Model file for the job. Use its own axes, mm. Round coordinates to 2 decimals unless told otherwise and drop trailing zeros. Use a Markdown table: item, result. Add a question column.
Q1. Cut at A-A (x = -32). State how many separate pieces and enclosed holes the cut face has, plus the area to 3 significant figures.
Q2. Pin check, flat tips, straight feed: pin 1 (0.6 mm diameter, centred on x = -60.5, y = 0.5, fed in from -Z) (3 decimals); pin 2 (0.5 mm diameter, centred on x = -20.5, y = -0.5, fed in from -Z); pin 3 (1 mm diameter, centred on y = -0.5, z = 17.5, fed in from -X). Stop position of each tip, or through.
Q3. Probe line 1 (X direction, y = 0.2, z = 0); line 2 (Z direction, x = -20.5, y = -1.8); line 3 (X direction, y = -1.55, z = 3.5). List the from-to ranges inside material, lowest first. Write a range as from..to.
from build123d import *

# Parameters (mm, degrees)
SKETCH1_R           = 12.7
BOSS_EXTRUDE1_DEPTH = 2.38125
CUT_EXTRUDE1_DEPTH  = 83.900304501
FILLET1_R           = 3.175
SKETCH3_RX          = 21.59
SKETCH3_RY          = 20.32
CUT_EXTRUDE2_DEPTH  = 83.900304501
CIRPATTERN1_COUNT   = 6
SKETCH4_R           = 1.27
CUT_EXTRUDE3_DEPTH  = 83.900304648
CIRPATTERN2_COUNT   = 6
BOSS_EXTRUDE2_DEPTH = 4.7625


with BuildPart() as part:
    # Sketch1 → Boss-Extrude1 (new, symmetric)
    with BuildSketch(Plane(origin=(0, 0, 0), x_dir=(1, 0, 0), z_dir=(0, 1, 0))):
        with BuildLine():
            Line((-60.1472, 5.553404471), (-60.1472, 9.525))
            Line((-60.1472, 9.525), (-38.322491971, 47.326503167))
            Line((-38.322491971, 47.326503167), (-34.88298935, 49.312300931))
            ThreePointArc((-34.88298935, 49.312300931), (-27.384375, 47.431128834), (-25.26421065, 54.865705402))
            Line((-25.26421065, 54.865705402), (-21.824708029, 56.851503167))
            Line((-21.824708029, 56.851503167), (21.824708029, 56.851503167))
            Line((21.824708029, 56.851503167), (25.26421065, 54.865705402))
            ThreePointArc((25.26421065, 54.865705402), (27.384375, 47.431128834), (34.88298935, 49.312300931))
            Line((34.88298935, 49.312300931), (38.322491971, 47.326503167))
            Line((38.322491971, 47.326503167), (60.1472, 9.525))
            Line((60.1472, 9.525), (60.1472, 5.553404471))
            ThreePointArc((60.1472, 5.553404471), (54.76875, 0), (60.1472, -5.553404471))
            Line((60.1472, -5.553404471), (60.1472, -9.525))
            Line((60.1472, -9.525), (38.322491971, -47.326503167))
            Line((38.322491971, -47.326503167), (34.88298935, -49.312300931))
            ThreePointArc((34.88298935, -49.312300931), (27.384375, -47.431128834), (25.26421065, -54.865705402))
            Line((25.26421065, -54.865705402), (21.824708029, -56.851503167))
            Line((21.824708029, -56.851503167), (-21.824708029, -56.851503167))
            Line((-21.824708029, -56.851503167), (-25.26421065, -54.865705402))
            ThreePointArc((-25.26421065, -54.865705402), (-27.384375, -47.431128834), (-34.88298935, -49.312300931))
            Line((-34.88298935, -49.312300931), (-38.322491971, -47.326503167))
            Line((-38.322491971, -47.326503167), (-60.1472, -9.525))
            Line((-60.1472, -9.525), (-60.1472, -5.553404471))
            ThreePointArc((-60.1472, -5.553404471), (-54.76875, 0), (-60.1472, 5.553404471))
        make_face()
        with Locations(Location((0, 0, 0), (0, 0, 90))):
            Circle(SKETCH1_R, mode=Mode.SUBTRACT)
    extrude(amount=BOSS_EXTRUDE1_DEPTH, both=True)

    # Sketch2 → Cut-Extrude1 (cut, through all)
    with BuildSketch(Plane(origin=(0, 2.38125, 0), x_dir=(1, 0, 0), z_dir=(0, 1, 0))):
        Polygon((10.61724051, -18.3896), (21.234481021, 0), (10.61724051, 18.3896), (-10.61724051, 18.3896), (-21.234481021, 0), (-10.61724051, -18.3896), align=None)
    extrude(amount=-CUT_EXTRUDE1_DEPTH, mode=Mode.SUBTRACT)

    # Fillet1
    fillet1_edges = [part.edges().sort_by_distance(p)[0] for p in [
        (10.61724051, 0, 18.3896),
        (-10.61724051, 0, 18.3896),
        (-21.234481021, 0, 0),
        (-10.61724051, 0, -18.3896),
        (10.61724051, 0, -18.3896),
        (21.234481021, 0, 0),
    ]]
    fillet(fillet1_edges, radius=FILLET1_R)

    # Sketch3 → Cut-Extrude2 (cut, through all)
    with BuildSketch(Plane(origin=(0, 2.38125, 0), x_dir=(1, 0, 0), z_dir=(0, 1, 0))):
        with Locations(Location((0, -56.851503167), (0, 0, -90))):
            Ellipse(SKETCH3_RX, SKETCH3_RY)
    cut_extrude2 = extrude(amount=-CUT_EXTRUDE2_DEPTH, mode=Mode.SUBTRACT)

    # CirPattern1: Cut-Extrude2 ×6 about axis
    cirpattern1_axis = Axis((0, -55, 0), (0, 1, 0))
    for i in range(1, CIRPATTERN1_COUNT):
        add(cut_extrude2.rotate(cirpattern1_axis, i * 360 / CIRPATTERN1_COUNT), mode=Mode.SUBTRACT)

    # Sketch4 → Cut-Extrude3 (cut, through all)
    with BuildSketch(Plane(origin=(0, 2.38125, 0), x_dir=(1, 0, 0), z_dir=(0, 1, 0))):
        with Locations(Location((45.212, 0, 0), (0, 0, 270))):
            Circle(SKETCH4_R)
    cut_extrude3 = extrude(amount=-CUT_EXTRUDE3_DEPTH, mode=Mode.SUBTRACT)

    # CirPattern2: Cut-Extrude3 ×6 about axis
    cirpattern2_axis = Axis((0, 0, 0), (0, 1, 0))
    for i in range(1, CIRPATTERN2_COUNT):
        add(cut_extrude3.rotate(cirpattern2_axis, i * 360 / CIRPATTERN2_COUNT), mode=Mode.SUBTRACT)

    # Sketch6 → Boss-Extrude2 (add)
    # profile 1 of 7: a face of its own
    with BuildSketch(Plane(origin=(0, 2.38125, 0), x_dir=(1, 0, 0), z_dir=(0, 1, 0))):
        with BuildLine():
            Line((11.533784063, -16.8021), (20.317937468, -1.5875))
            ThreePointArc((20.317937468, -1.5875), (20.743306811, 0), (20.317937468, 1.5875))
            Line((20.317937468, 1.5875), (11.533784063, 16.8021))
            ThreePointArc((11.533784063, 16.8021), (10.371653406, 17.964230657), (8.784153406, 18.3896))
            Line((8.784153406, 18.3896), (-8.784153406, 18.3896))
            ThreePointArc((-8.784153406, 18.3896), (-10.371653406, 17.964230657), (-11.533784063, 16.8021))
            Line((-11.533784063, 16.8021), (-20.317937468, 1.5875))
            ThreePointArc((-20.317937468, 1.5875), (-20.743306811, 0), (-20.317937468, -1.5875))
            Line((-20.317937468, -1.5875), (-11.533784063, -16.8021))
            ThreePointArc((-11.533784063, -16.8021), (-10.371653406, -17.964230657), (-8.784153406, -18.3896))
            Line((-8.784153406, -18.3896), (8.784153406, -18.3896))
            ThreePointArc((8.784153406, -18.3896), (10.371653406, -17.964230657), (11.533784063, -16.8021))
        make_face()
        with BuildLine():
            Line((19.658026111, 1.2065), (10.873872705, 16.4211))
            ThreePointArc((10.873872705, 16.4211), (9.990653406, 17.304319299), (8.784153406, 17.6276))
            Line((8.784153406, 17.6276), (-8.784153406, 17.6276))
            ThreePointArc((-8.784153406, 17.6276), (-9.990653406, 17.304319299), (-10.873872705, 16.4211))
            Line((-10.873872705, 16.4211), (-19.658026111, 1.2065))
            ThreePointArc((-19.658026111, 1.2065), (-19.981306811, 0), (-19.658026111, -1.2065))
            Line((-19.658026111, -1.2065), (-10.873872705, -16.4211))
            ThreePointArc((-10.873872705, -16.4211), (-9.990653406, -17.304319299), (-8.784153406, -17.6276))
            Line((-8.784153406, -17.6276), (8.784153406, -17.6276))
            ThreePointArc((8.784153406, -17.6276), (9.990653406, -17.304319299), (10.873872705, -16.4211))
            Line((10.873872705, -16.4211), (19.658026111, -1.2065))
            ThreePointArc((19.658026111, -1.2065), (19.981306811, 0), (19.658026111, 1.2065))
        make_face(mode=Mode.SUBTRACT)
    # profile 2 of 7: a face of its own
    with BuildSketch(Plane(origin=(0, 2.38125, 0), x_dir=(1, 0, 0), z_dir=(0, 1, 0))):
        with BuildLine():
            Line((-60.1472, -5.553404471), (-60.1472, -9.525))
            Line((-60.1472, -9.525), (-60.9092, -9.525))
            Line((-60.9092, -9.525), (-60.9092, -4.75852324))
            ThreePointArc((-60.9092, -4.75852324), (-55.53075, 0), (-60.9092, 4.75852324))
            Line((-60.9092, 4.75852324), (-60.9092, 9.525))
            Line((-60.9092, 9.525), (-60.1472, 9.525))
            Line((-60.1472, 9.525), (-60.1472, 5.553404471))
            ThreePointArc((-60.1472, 5.553404471), (-54.76875, 0), (-60.1472, -5.553404471))
        make_face()
    # profile 3 of 7: a face of its own
    with BuildSketch(Plane(origin=(0, 2.38125, 0), x_dir=(1, 0, 0), z_dir=(0, 1, 0))):
        with BuildLine():
            Line((-34.88298935, 49.312300931), (-38.322491971, 47.326503167))
            Line((-38.322491971, 47.326503167), (-38.703491971, 47.986414524))
            Line((-38.703491971, 47.986414524), (-34.57560201, 50.369652904))
            ThreePointArc((-34.57560201, 50.369652904), (-27.765375, 48.091040191), (-26.33359799, 55.128176144))
            Line((-26.33359799, 55.128176144), (-22.205708029, 57.511414524))
            Line((-22.205708029, 57.511414524), (-21.824708029, 56.851503167))
            Line((-21.824708029, 56.851503167), (-25.26421065, 54.865705402))
            ThreePointArc((-25.26421065, 54.865705402), (-27.384375, 47.431128834), (-34.88298935, 49.312300931))
        make_face()
    # profile 4 of 7: a face of its own
    with BuildSketch(Plane(origin=(0, 2.38125, 0), x_dir=(1, 0, 0), z_dir=(0, 1, 0))):
        with BuildLine():
            Line((25.26421065, 54.865705402), (21.824708029, 56.851503167))
            Line((21.824708029, 56.851503167), (22.205708029, 57.511414524))
            Line((22.205708029, 57.511414524), (26.33359799, 55.128176144))
            ThreePointArc((26.33359799, 55.128176144), (27.765375, 48.091040191), (34.57560201, 50.369652904))
            Line((34.57560201, 50.369652904), (38.703491971, 47.986414524))
            Line((38.703491971, 47.986414524), (38.322491971, 47.326503167))
            Line((38.322491971, 47.326503167), (34.88298935, 49.312300931))
            ThreePointArc((34.88298935, 49.312300931), (27.384375, 47.431128834), (25.26421065, 54.865705402))
        make_face()
    # profile 5 of 7: a face of its own
    with BuildSketch(Plane(origin=(0, 2.38125, 0), x_dir=(1, 0, 0), z_dir=(0, 1, 0))):
        with BuildLine():
            Line((60.1472, 5.553404471), (60.1472, 9.525))
            Line((60.1472, 9.525), (60.9092, 9.525))
            Line((60.9092, 9.525), (60.9092, 4.75852324))
            ThreePointArc((60.9092, 4.75852324), (55.53075, 0), (60.9092, -4.75852324))
            Line((60.9092, -4.75852324), (60.9092, -9.525))
            Line((60.9092, -9.525), (60.1472, -9.525))
            Line((60.1472, -9.525), (60.1472, -5.553404471))
            ThreePointArc((60.1472, -5.553404471), (54.76875, 0), (60.1472, 5.553404471))
        make_face()
    # profile 6 of 7: a face of its own
    with BuildSketch(Plane(origin=(0, 2.38125, 0), x_dir=(1, 0, 0), z_dir=(0, 1, 0))):
        with BuildLine():
            Line((34.88298935, -49.312300931), (38.322491971, -47.326503167))
            Line((38.322491971, -47.326503167), (38.703491971, -47.986414524))
            Line((38.703491971, -47.986414524), (34.57560201, -50.369652904))
            ThreePointArc((34.57560201, -50.369652904), (27.765375, -48.091040191), (26.33359799, -55.128176144))
            Line((26.33359799, -55.128176144), (22.205708029, -57.511414524))
            Line((22.205708029, -57.511414524), (21.824708029, -56.851503167))
            Line((21.824708029, -56.851503167), (25.26421065, -54.865705402))
            ThreePointArc((25.26421065, -54.865705402), (27.384375, -47.431128834), (34.88298935, -49.312300931))
        make_face()
    # profile 7 of 7: a face of its own
    with BuildSketch(Plane(origin=(0, 2.38125, 0), x_dir=(1, 0, 0), z_dir=(0, 1, 0))):
        with BuildLine():
            Line((-25.26421065, -54.865705402), (-21.824708029, -56.851503167))
            Line((-21.824708029, -56.851503167), (-22.205708029, -57.511414524))
            Line((-22.205708029, -57.511414524), (-26.33359799, -55.128176144))
            ThreePointArc((-26.33359799, -55.128176144), (-27.765375, -48.091040191), (-34.57560201, -50.369652904))
            Line((-34.57560201, -50.369652904), (-38.703491971, -47.986414524))
            Line((-38.703491971, -47.986414524), (-38.322491971, -47.326503167))
            Line((-38.322491971, -47.326503167), (-34.88298935, -49.312300931))
            ThreePointArc((-34.88298935, -49.312300931), (-27.384375, -47.431128834), (-25.26421065, -54.865705402))
        make_face()
    extrude(amount=-BOSS_EXTRUDE2_DEPTH)


solid = part.part
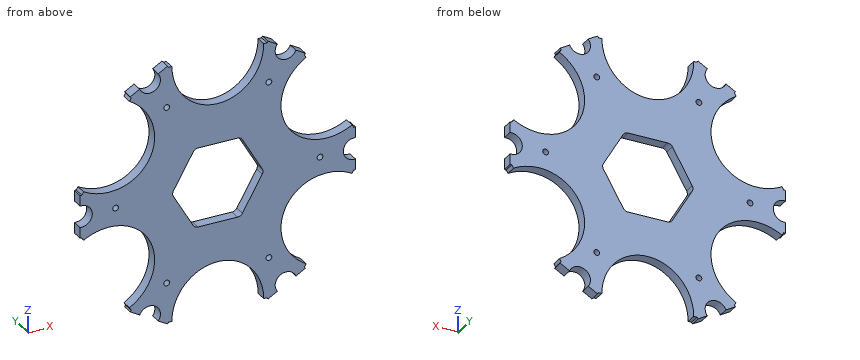
Checked values:
| question | item | result |
|---|---|---|
| 1 | separate pieces | 3 |
| 1 | enclosed holes | 0 |
| 1 | area | 225 mm^2 |
| 2 | pin 1 | stops at z = -9.525 |
| 2 | pin 2 | stops at z = -56.85 |
| 2 | pin 3 | stops at x = -30.92 |
| 3 | line 1 | x = -55.53..-46.48, -43.94..-19.98, 19.98..43.94, 46.48..55.53 |
| 3 | line 2 | z = -56.85..56.85 |
| 3 | line 3 | x = -57.05..-18.33, 18.33..57.05 |
